Geometry: final body of the model. Coordinates: model frame, mm. A direction names the side the tool comes from. Give positions to 0.01 mm unless a question says otherwise; leave off trailing zeros. Write each loop counter-clockwise with the first axis right and the second up, starting at its lowest first coordinate (ties: lowest second). Pieces come first, ordered by that corner, then holes. Notation, with made-up numbers: M -34,42.5 L -20,42.5 A25 ccw -20,57.5 Z; hole C 77.25,67 d11. An arc over 180 degrees is marked long. Use a Markdown table: item, result. Add a question column.
1) Line query: line 1 (X direction, y = -2.45, z = 18); line 2 (Z direction, x = 32.45, y = 106.15) (3 decimals); line 3 (Z direction, x = 20.5, y = 65.5). Output: solid intervals per line, ascending.
2) Section C-C on x = 20. Return the cut outline in (y, z).
3) Section B-B on z = 0. Return the cut outline in (x, y), then the cut area to 3 significant figures.
4) Draft query along Y for faces 5 (the cylindrical face through (32.36, 104.72, -5.22)), 6 (the cylindrical face through (29.03, 0.9, -12.36)), 7 (the flat face through (34.393, 96, 0)), 8 (the flat face through (30.393, 104.6, 6.4)). Return one class per face: +Y half, -Y half, draft (parallel to the pull), parting line (faces both ways), or undercut.
5) Section A-A on z = -18. Return the cut outline in (x, y), then the cut area to 3 significant figures.
6) Section D-D on x = 27.5. Return the cut outline in (y, z).
7) Pin query (flat end, axial travel): pin 1 (8 mm diameter, centred on x = 22.5, z = -5, fed in from +Y); pin 2 (5 mm diameter, centred on y = 93.5, z = -8.5, fed in from -X); pin 3 (3 mm diameter, centred on x = 31.5, y = 108.5, fed in from +Z); pin 4 (4 mm diameter, centred on x = 7.25, z = 18, fed in from -Y). Return the tip coordinate at first contact, or that it passes through.
8) Set-up query: faces 1 (the flat face through (30, 96, 8.85)), 2 (the flat face through (47.787, 100, 0)), 3 (the flat face through (12.75, 61.21, 0.11)), 4 (the cylindrical face through (32.892, 106.061, -0.055)). Return all of +Z, -Z, +X, -X, +Y, -Y with unobstructed straight access to the full face (end or side cutting, diameter ignored); none if empty.
```python
from build123d import *

# Parameters (mm, degrees)
BOSS_EXTRUDE1_DEPTH     = 11.5
SKETCH2_OUTSIDE_W       = 84.912
SKETCH2_OUTSIDE_H       = 140.162
CUT_EXTRUDE2_DEPTH      = 7.5
CUT_EXTRUDE3_DEPTH      = 129.307516771
CUT_EXTRUDE3_DEPTH_BACK = 129.307516771
SKETCH4_R               = 1.75
SKETCH5_W               = 57.250055546
SKETCH5_H               = 43
BOSS_EXTRUDE2_DEPTH     = 4
SKETCH6_R               = 1.75
CUT_EXTRUDE4_DEPTH      = 129.047135306
FILLET1_R               = 3
SKETCH7_R               = 5.08
BOSS_EXTRUDE3_DEPTH     = 10
SKETCH11_W              = 13
SKETCH11_H              = 17.7
CUT_EXTRUDE7_DEPTH      = 20
SKETCH8_W               = 4
SKETCH8_H               = 12.7
BOSS_EXTRUDE4_DEPTH     = 8.85
SKETCH9_R               = 2.5
CUT_EXTRUDE5_DEPTH      = 116.967836159
SKETCH10_R              = 1.5
CUT_EXTRUDE6_DEPTH      = 4


with BuildPart() as part:
    # Sketch1 → Boss-Extrude1 (new, symmetric)
    with BuildSketch(Plane.XY):
        Polygon((0, 45), (0, 0), (57.250055546, 0), (57.250055546, 15), (24.066011022, 34.158817039), (46.210390637, 95), (57.250055546, 112.5), (34.392967841, 112.5), align=None)
    extrude(amount=BOSS_EXTRUDE1_DEPTH, both=True)

    # Sketch2 outside → Cut-Extrude2 (cut, symmetric)
    with BuildSketch(Plane.XY):
        with Locations((28.625, 56.25)):
            Rectangle(SKETCH2_OUTSIDE_W, SKETCH2_OUTSIDE_H)
        Polygon((4, 44.039684964), (21.742887775, 78.862062909), (47.787485624, 102.92976146), (47.787485624, 97.5), (57.250055546, 112.5), (52.250055546, 112.5), (18.50330035, 81.314771653), (0, 45), (0, 0), (57.250055546, 0), (57.250055546, 6.97368477), (4, 24.475940791), align=None, mode=Mode.SUBTRACT)
        Polygon((18.50330035, 81.314771653), (52.250055546, 112.5), (34.392967841, 112.5), align=None, mode=Mode.SUBTRACT)
    extrude(amount=CUT_EXTRUDE2_DEPTH, both=True, mode=Mode.SUBTRACT)

    # Sketch4 → Cut-Extrude3 (cut, two sides: drawn at the far end of the back side and taken through both)
    with BuildSketch(Plane.XY.offset(11.5).offset(-CUT_EXTRUDE3_DEPTH_BACK)):
        with Locations((45.250055546, 16.444166257)):
            Circle(SKETCH4_R)
        with Locations((31.000040397, 21.127868666)):
            Circle(SKETCH4_R)
        with Locations((16.750025248, 25.811571075)):
            Circle(SKETCH4_R)
    extrude(amount=CUT_EXTRUDE3_DEPTH + CUT_EXTRUDE3_DEPTH_BACK, mode=Mode.SUBTRACT)

    # Sketch5 → Boss-Extrude2 (add)
    with BuildSketch(Plane.XZ):
        with Locations((28.625027773, 0)):
            Rectangle(SKETCH5_W, SKETCH5_H)
    extrude(amount=BOSS_EXTRUDE2_DEPTH)

    # Sketch6 → Cut-Extrude4 (cut, symmetric)
    with BuildSketch(Plane(origin=(0, 0, 0), x_dir=(1, 0, 0), z_dir=(0, 1, 0))):
        with Locations(Location((7.250055546, 18, 0), (0, 0, 270))):
            Circle(SKETCH6_R)
        with Locations(Location((47.250055546, 18, 0), (0, 0, 270))):
            Circle(SKETCH6_R)
    cut_extrude4 = extrude(amount=CUT_EXTRUDE4_DEPTH, both=True, mode=Mode.SUBTRACT)

    # Mirror5: Cut-Extrude4 across plane
    add(cut_extrude4.mirror(Plane.XY), mode=Mode.SUBTRACT)

    # Fillet1
    fillet1_edges = [part.edges().sort_by_distance(p)[0] for p in [
        (28.625027773, 0, 11.5),
        (28.625027773, 0, -11.5),
    ]]
    fillet(fillet1_edges, radius=FILLET1_R)

    # Sketch7 → Boss-Extrude3 (add)
    with BuildSketch(Plane(origin=(0, 112.5, 0), x_dir=(1, 0, 0), z_dir=(0, 1, 0))):
        with Locations(Location((47.000055546, 0, 0), (0, 0, 270))):
            Circle(SKETCH7_R)
    extrude(amount=BOSS_EXTRUDE3_DEPTH)

    # Sketch11 → Cut-Extrude7 (cut)
    with BuildSketch(Plane(origin=(0, 112.5, 0), x_dir=(1, 0, 0), z_dir=(0, 1, 0))):
        with Locations((27.892967841, 0)):
            Rectangle(SKETCH11_W, SKETCH11_H)
    extrude(amount=-CUT_EXTRUDE7_DEPTH, mode=Mode.SUBTRACT)

    # Sketch8 → Boss-Extrude4 (add, symmetric)
    with BuildSketch(Plane.XY):
        with Locations((32.392967841, 106.15)):
            Rectangle(SKETCH8_W, SKETCH8_H)
    extrude(amount=BOSS_EXTRUDE4_DEPTH, both=True)

    # Sketch9 → Cut-Extrude5 (cut, through all)
    with BuildSketch(Plane(origin=(47.030298994, 99.8, 0), x_dir=(-1, 0, 0), z_dir=(0, -1, 0))):
        with Locations((16.637331153, 0)):
            Circle(SKETCH9_R)
    extrude(amount=-CUT_EXTRUDE5_DEPTH, mode=Mode.SUBTRACT)

    # Sketch10 → Cut-Extrude6 (cut)
    with BuildSketch(Plane(origin=(30.392967841, -1.431684556, 0), x_dir=(0, 0, 1), z_dir=(-1, 0, 0))):
        with Locations(Location((-5.675, 107.581684556, 0), (0, 0, 270))):
            Circle(SKETCH10_R)
        with Locations(Location((5.675, 107.581684556, 0), (0, 0, 270))):
            Circle(SKETCH10_R)
    extrude(amount=-CUT_EXTRUDE6_DEPTH, mode=Mode.SUBTRACT)


solid = part.part
```
Found:
| question | item | result |
|---|---|---|
| 1 | line 1 | 0 to 5.5, 9 to 45.5, 49 to 57.25 |
| 1 | line 2 | -11.5 to -7.175, -4.175 to -1.421, 1.421 to 4.175, 7.175 to 11.5 |
| 1 | line 3 | -11.5 to -7.5, 7.5 to 11.5 |
| 2 | outline | M -4,-21.5 L 0,-21.5 L 0,-14.5 A3 cw 3,-11.5 L 84.25,-11.5 L 84.25,11.5 L 3,11.5 A3 cw 0,14.5 L 0,21.5 L -4,21.5 Z; hole M 19.22,-7.5 L 75.44,-7.5 L 75.44,7.5 L 19.22,7.5 Z |
| 3 | outline | M 0,-4 L 57.25,-4 L 57.25,6.97 L 4,24.48 L 4,44.04 L 21.74,78.86 L 47.79,102.93 L 47.79,97.5 L 57.25,112.5 L 52.08,112.5 L 52.08,122.5 L 41.92,122.5 L 41.92,112.5 L 32.89,112.5 L 32.89,99.8 L 34.39,99.8 L 34.39,92.5 L 24.2,92.5 L 0,45 Z |
| 3 | area | 1,910 mm² |
| 4 | face 5 | undercut |
| 4 | face 6 | +Y half |
| 4 | face 7 | undercut |
| 4 | face 8 | draft |
| 5 | outline | M 0,-4 L 5.5,-4 L 5.5,0 L 0,0 Z; M 9,-4 L 45.5,-4 L 45.5,0 L 9,0 Z; M 49,-4 L 57.25,-4 L 57.25,0 L 49,0 Z |
| 5 | area | 201 mm² |
| 6 | outline | M -4,-21.5 L 0,-21.5 L 0,-14.5 A3 cw 3,-11.5 L 32.18,-11.5 L 32.18,-7.5 L 16.75,-7.5 L 16.75,7.5 L 32.18,7.5 L 32.18,11.5 L 3,11.5 A3 cw 0,14.5 L 0,21.5 L -4,21.5 Z; M 43.59,-11.5 L 98.97,-11.5 L 98.97,-8.85 L 92.5,-8.85 L 92.5,8.85 L 98.97,8.85 L 98.97,11.5 L 43.59,11.5 L 43.59,7.5 L 84.18,7.5 L 84.18,-7.5 L 43.59,-7.5 Z |
| 7 | pin 1 | y = 92.5 |
| 7 | pin 2 | x = 23.44 |
| 7 | pin 3 | z = 11.5 |
| 7 | pin 4 | y = -4 |
| 8 | face 1 | -X |
| 8 | face 2 | none |
| 8 | face 3 | +X |
| 8 | face 4 | -X, +Y |
